Build history of the part. All positions in model axes, mm. Coordinates: 2 decimals unless noted, no trailing zeros. Order: outer loops, then holes, each group sorted by start corner. A loop starts at its lowest first (then second) coordinate and runs counter-clockwise, first axis right, second up. Notation, with made-up numbers: (5.25, 89.5) - (53.25, 89.5) arc R21 cw to (53.25, 103.5) - close; hole circle Ø11 at (79, -10). An arc over 180 degrees is marked (long way). One line per item, written item: value.
from build123d import *

# Parameters (mm, degrees)
F0_W     = 10.5
F0_H     = 28.32
F1_DEPTH = 1
F3_DEPTH = 1.5
F4_SIZE  = 3


with BuildPart() as f1:
    # F0 (on Top) → F1 (new body)
    with BuildSketch(Plane.XY):
        Rectangle(F0_W, F0_H)
    extrude(amount=F1_DEPTH)

    # F2 (on face) → F3 (cut)
    with BuildSketch(Plane.XY.offset(1)):
        with BuildLine():
            ThreePointArc((2.5, 8.79), (-1.767766953, 10.557766953), (0, 6.29))
            ThreePointArc((0, 6.29), (1.767766953, 7.022233047), (2.5, 8.79))
        make_face()
        with BuildLine():
            ThreePointArc((0, -0.19), (-2.5, -2.69), (0, -5.19))
            ThreePointArc((0, -5.19), (1.767766953, -4.457766953), (2.5, -2.69))
            ThreePointArc((2.5, -2.69), (1.767766953, -0.922233047), (0, -0.19))
        make_face()
    extrude(amount=-F3_DEPTH, mode=Mode.SUBTRACT)

    # F4
    f4_edges = [f1.edges().sort_by_distance(p)[0] for p in [
        (-5.25, -14.16, 0.5),
    ]]
    chamfer(f4_edges, length=F4_SIZE)


solid = f1.part
1. Band-saw the part on D-D, the plane x = -4.5. Give the cut face in (y, z).
Values found:
outline: (-11.91, 0) - (14.16, 0) - (14.16, 1) - (-11.91, 1) - close
2. Probe line 1 along Y through (x, z) = (0, 0.8); line 2 along X through (y, z) = (8.79, 0.5); line 3 along Y through (x, z) = (1.25, 0.35). List the from-to ranges inside material, lowest first.
Values found:
line 1: y = -14.16 to -5.19, -0.19 to 6.29, 11.29 to 14.16
line 2: x = -5.25 to -2.5, 2.5 to 5.25
line 3: y = -14.16 to -4.86, -0.52 to 6.62, 10.96 to 14.16
3. Band-saw the part on B-B, the plane z = 0.7. Give the cut face in (x, y), and give its area (3 significant figures).
Values found:
outline: (-5.25, -11.16) - (-2.25, -14.16) - (5.25, -14.16) - (5.25, 14.16) - (-5.25, 14.16) - close; hole circle Ø5 at (0, -2.69); hole circle Ø5 at (0, 8.79)
area: 254 mm2
4. Band-saw the part on C-C, the plane y = -2.25. Give the cut face in (x, z), and give its area (3 significant figures).
Values found:
outline: (-5.25, 0) - (-2.46, 0) - (-2.46, 1) - (-5.25, 1) - close; (2.46, 0) - (5.25, 0) - (5.25, 1) - (2.46, 1) - close
area: 5.58 mm2
5. Band-saw the part on A-A, the plane x = -2. Give the cut face in (y, z).
Values found:
outline: (-14.16, 0) - (-4.19, 0) - (-4.19, 1) - (-14.16, 1) - close; (-1.19, 0) - (7.29, 0) - (7.29, 1) - (-1.19, 1) - close; (10.29, 0) - (14.16, 0) - (14.16, 1) - (10.29, 1) - close
